```python
from build123d import *

# Parameters (mm, degrees)
SKETCH1_W           = 25
SKETCH1_H           = 30
BOSS_EXTRUDE1_DEPTH = 2.5
SKETCH3_W           = 25
SKETCH3_H           = 30
SKETCH3_W_2         = 20
SKETCH3_H_2         = 21
BOSS_EXTRUDE2_DEPTH = 2.5
SKETCH5_R           = 5
CUT_EXTRUDE1_DEPTH  = 2.5
FILLET2_R           = 2
SKETCH6_W           = 19.4
SKETCH6_H           = 2.5
BOSS_EXTRUDE4_DEPTH = 2.5


with BuildPart() as part:
    # Sketch1 → Boss-Extrude1 (new body)
    with BuildSketch(Plane(origin=(0, 0, 0), x_dir=(1, 0, 0), z_dir=(0, 1, 0))):
        Rectangle(SKETCH1_W, SKETCH1_H)
    extrude(amount=BOSS_EXTRUDE1_DEPTH)

    # Sketch3 → Boss-Extrude2 (add)
    with BuildSketch(Plane(origin=(0, 2.5, 0), x_dir=(1, 0, 0), z_dir=(0, 1, 0))):
        Rectangle(SKETCH3_W, SKETCH3_H)
        with Locations((0, 2)):
            Rectangle(SKETCH3_W_2, SKETCH3_H_2, mode=Mode.SUBTRACT)
    extrude(amount=BOSS_EXTRUDE2_DEPTH)

    # Sketch5 → Cut-Extrude1 (cut)
    with BuildSketch(Plane(origin=(0, 2.5, 0), x_dir=(1, 0, 0), z_dir=(0, 1, 0))):
        with Locations(Location((0, 5, 0), (0, 0, 270))):  # turned: the seam where the file's is
            Circle(SKETCH5_R)
    extrude(amount=-CUT_EXTRUDE1_DEPTH, mode=Mode.SUBTRACT)

    # Fillet2
    fillet2_edges = [part.edges().sort_by_distance(p)[0] for p in [
        (0, 0, 15),
        (-12.5, 0, 0),
        (0, 0, -15),
        (12.5, 0, 0),
        (12.5, 2.5, 15),
        (-12.5, 2.5, 15),
        (-12.5, 2.5, -15),
        (12.5, 2.5, -15),
    ]]
    fillet(fillet2_edges, radius=FILLET2_R)

    # Sketch6 → Boss-Extrude4 (add)
    with BuildSketch(Plane(origin=(0, 5, 0), x_dir=(1, 0, 0), z_dir=(0, 1, 0))):
        with Locations((0, -9.75)):
            Rectangle(SKETCH6_W, SKETCH6_H)
    extrude(amount=BOSS_EXTRUDE4_DEPTH)


solid = part.part
```
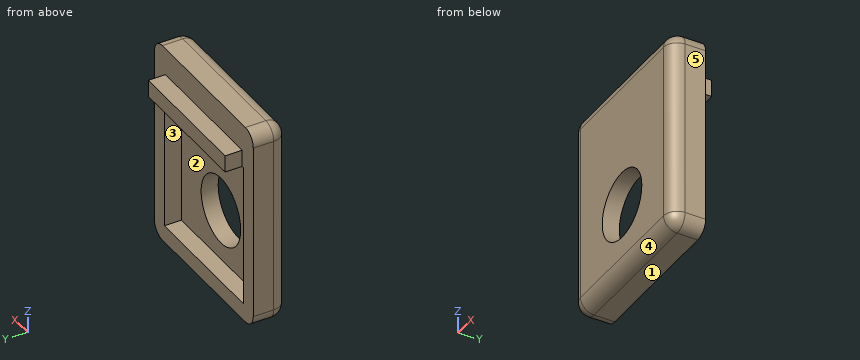
Work out the finished part from the listing and answer in its coordinate system (mm). Face numbers are marked on the shaded views. A direction names the side the tool comes from. Give positions to 0.01 mm unless a question says otherwise; leave off trailing zeros. Loops run counter-clockwise (first coordinate to the right, second up) from the corner with the lowest first, then second, coordinate; pieces in that order, holes last. Notation, with made-up numbers: (74.25, 19.25) -> (112.25, 19.25) arc R22 cw to (112.25, 44.25) -> close; hole circle Ø1 at (-26, 83.25). An arc over 180 degrees is marked (long way). Put each result on its own line as item: value. Start each with the question number.
Item 1: The part is cut by section C-C (z = -5). Give the vertices of the cut face in (x, y), then the cut area to 3 significant figures.
Item 2: The part is cut by section A-A (x = 0). Give the vertices of the cut face in (y, z), then the cut area to 3 significant figures.
Item 3: Find the intervals of material crossed by L1, parallel to X at y = 4, z = -5; L2, parallel to Z at x = -9, y = 4.5; L3, parallel to Z at x = -0.25, y = 2, in increasing order. Write a range as [from, to].
Item 4: Each of these flat-tipped pins is pushed along its axis until it touches: P1, Ø10, axis at x = 0, z = 0.5, coming from the +Y side; P2, Ø0.8, axis at x = 2.5, y = 6.5, coming from the +Z side. Where does it stop, or does it pass through?
Item 5: The part is cut by section B-B (y = 4.5). Give the vertices of the cut face in (x, z).
Item 6: The mould has two halves that part along X. Classify the marked faces 3, 4 and 5: released by +X, released by -X, zero draft, split by the parting line, or undercut.
Item 7: The part is cut by section D-D (z = 1.75). Give the vertices of the cut face in (x, y), then the cut area to 3 significant figures.
Item 8: Which of the six approach directions +Z, -Z, +X, -X, +Y, -Y give full straight-line access (tool end or side, diameter ignored) to the marked faces 1 and 2?
Answers below:
1. outline: (-12.5, 2) arc R2 ccw to (-10.5, 0) -> (-5, 0) -> (-5, 2.5) -> (-10, 2.5) -> (-10, 5) -> (-12.5, 5) -> close; (5, 0) -> (10.5, 0) arc R2 ccw to (12.5, 2) -> (12.5, 5) -> (10, 5) -> (10, 2.5) -> (5, 2.5) -> close
1. area: 48.3 mm2
2. outline: (0, -13) arc R2 ccw to (2, -15) -> (5, -15) -> (5, -12.5) -> (2.5, -12.5) -> (2.5, -10) -> (0, -10) -> close; (0, 0) -> (2.5, 0) -> (2.5, 8.5) -> (7.5, 8.5) -> (7.5, 11) -> (5, 11) -> (5, 15) -> (2, 15) arc R2 ccw to (0, 13) -> close
2. area: 77.0 mm2
3. L1: [-12.5, -10], [10, 12.5]
3. L2: [-15, -12.5], [8.5, 15]
3. L3: [-15, -9.99], [-0.01, 15]
4. P1: y = 2.5
4. P2: z = 11
5. outline: (-12.5, -13) arc R2 ccw to (-10.5, -15) -> (10.5, -15) arc R2 ccw to (12.5, -13) -> (12.5, 13) arc R2 ccw to (10.5, 15) -> (-10.5, 15) arc R2 ccw to (-12.5, 13) -> close; hole (-10, -12.5) -> (10, -12.5) -> (10, 8.5) -> (-10, 8.5) -> close
6. face 3: undercut
6. face 4: zero draft
6. face 5: released by +X
7. outline: (-12.5, 2) arc R2 ccw to (-10.5, 0) -> (10.5, 0) arc R2 ccw to (12.5, 2) -> (12.5, 5) -> (10, 5) -> (10, 2.5) -> (-10, 2.5) -> (-10, 5) -> (-12.5, 5) -> close
7. area: 73.3 mm2
8. face 1: -Z, +X, -X, +Y, -Y
8. face 2: +Y
